```python
from build123d import *

# Parameters (mm, degrees)
MODEL_R             = 95.25
MODEL_R_2           = 85.725
MODEL_R_3           = 1.6724
BOSS_EXTRUDE1_DEPTH = 4


with BuildPart() as part:
    # Model → Boss-Extrude1 (new body)
    with BuildSketch(Plane.XY):
        Circle(MODEL_R)
        Circle(MODEL_R_2, mode=Mode.SUBTRACT)
        with Locations((90.208557236, -7.099567425)):
            Circle(MODEL_R_3, mode=Mode.SUBTRACT)
        with Locations((89.37344872, -14.155363655)):
            Circle(MODEL_R_3, mode=Mode.SUBTRACT)
        with Locations((87.987323172, -21.123887362)):
            Circle(MODEL_R_3, mode=Mode.SUBTRACT)
        with Locations((86.058726518, -27.962175279)):
            Circle(MODEL_R_3, mode=Mode.SUBTRACT)
        with Locations((83.599549198, -34.628067086)):
            Circle(MODEL_R_3, mode=Mode.SUBTRACT)
        with Locations((80.624952857, -41.080465345)):
            Circle(MODEL_R_3, mode=Mode.SUBTRACT)
        with Locations((77.153276872, -47.279588875)):
            Circle(MODEL_R_3, mode=Mode.SUBTRACT)
        with Locations((73.205925279, -53.187218017)):
            Circle(MODEL_R_3, mode=Mode.SUBTRACT)
        with Locations((68.807234812, -58.766930273)):
            Circle(MODEL_R_3, mode=Mode.SUBTRACT)
        with Locations((63.984324863, -63.984324863)):
            Circle(MODEL_R_3, mode=Mode.SUBTRACT)
        with Locations((58.766930273, -68.807234812)):
            Circle(MODEL_R_3, mode=Mode.SUBTRACT)
        with Locations((53.187218017, -73.205925279)):
            Circle(MODEL_R_3, mode=Mode.SUBTRACT)
        with Locations((47.279588875, -77.153276872)):
            Circle(MODEL_R_3, mode=Mode.SUBTRACT)
        with Locations((41.080465345, -80.624952857)):
            Circle(MODEL_R_3, mode=Mode.SUBTRACT)
        with Locations((34.628067086, -83.599549198)):
            Circle(MODEL_R_3, mode=Mode.SUBTRACT)
        with Locations((27.962175279, -86.058726518)):
            Circle(MODEL_R_3, mode=Mode.SUBTRACT)
        with Locations((21.123887362, -87.987323172)):
            Circle(MODEL_R_3, mode=Mode.SUBTRACT)
        with Locations((14.155363655, -89.37344872)):
            Circle(MODEL_R_3, mode=Mode.SUBTRACT)
        with Locations((7.099567425, -90.208557236)):
            Circle(MODEL_R_3, mode=Mode.SUBTRACT)
        with Locations((0, -90.4875)):
            Circle(MODEL_R_3, mode=Mode.SUBTRACT)
        with Locations((-7.099567425, -90.208557236)):
            Circle(MODEL_R_3, mode=Mode.SUBTRACT)
        with Locations((-14.155363655, -89.37344872)):
            Circle(MODEL_R_3, mode=Mode.SUBTRACT)
        with Locations((-21.123887362, -87.987323172)):
            Circle(MODEL_R_3, mode=Mode.SUBTRACT)
        with Locations((-27.962175279, -86.058726518)):
            Circle(MODEL_R_3, mode=Mode.SUBTRACT)
        with Locations((-34.628067086, -83.599549198)):
            Circle(MODEL_R_3, mode=Mode.SUBTRACT)
        with Locations((-41.080465345, -80.624952857)):
            Circle(MODEL_R_3, mode=Mode.SUBTRACT)
        with Locations((-47.279588875, -77.153276872)):
            Circle(MODEL_R_3, mode=Mode.SUBTRACT)
        with Locations((-53.187218017, -73.205925279)):
            Circle(MODEL_R_3, mode=Mode.SUBTRACT)
        with Locations((-58.766930273, -68.807234812)):
            Circle(MODEL_R_3, mode=Mode.SUBTRACT)
        with Locations((-63.984324863, -63.984324863)):
            Circle(MODEL_R_3, mode=Mode.SUBTRACT)
        with Locations((-68.807234812, -58.766930273)):
            Circle(MODEL_R_3, mode=Mode.SUBTRACT)
        with Locations((-73.205925279, -53.187218017)):
            Circle(MODEL_R_3, mode=Mode.SUBTRACT)
        with Locations((-77.153276872, -47.279588875)):
            Circle(MODEL_R_3, mode=Mode.SUBTRACT)
        with Locations((-80.624952857, -41.080465345)):
            Circle(MODEL_R_3, mode=Mode.SUBTRACT)
        with Locations((-83.599549198, -34.628067086)):
            Circle(MODEL_R_3, mode=Mode.SUBTRACT)
        with Locations((-86.058726518, -27.962175279)):
            Circle(MODEL_R_3, mode=Mode.SUBTRACT)
        with Locations((-87.987323172, -21.123887362)):
            Circle(MODEL_R_3, mode=Mode.SUBTRACT)
        with Locations((-89.37344872, -14.155363655)):
            Circle(MODEL_R_3, mode=Mode.SUBTRACT)
        with Locations((-90.208557236, -7.099567425)):
            Circle(MODEL_R_3, mode=Mode.SUBTRACT)
        with Locations((-90.4875, 0)):
            Circle(MODEL_R_3, mode=Mode.SUBTRACT)
        with Locations((-90.208557236, 7.099567425)):
            Circle(MODEL_R_3, mode=Mode.SUBTRACT)
        with Locations((-89.37344872, 14.155363655)):
            Circle(MODEL_R_3, mode=Mode.SUBTRACT)
        with Locations((-87.987323172, 21.123887362)):
            Circle(MODEL_R_3, mode=Mode.SUBTRACT)
        with Locations((-86.058726518, 27.962175279)):
            Circle(MODEL_R_3, mode=Mode.SUBTRACT)
        with Locations((-83.599549198, 34.628067086)):
            Circle(MODEL_R_3, mode=Mode.SUBTRACT)
        with Locations((-80.624952857, 41.080465345)):
            Circle(MODEL_R_3, mode=Mode.SUBTRACT)
        with Locations((-77.153276872, 47.279588875)):
            Circle(MODEL_R_3, mode=Mode.SUBTRACT)
        with Locations((-73.205925279, 53.187218017)):
            Circle(MODEL_R_3, mode=Mode.SUBTRACT)
        with Locations((-68.807234812, 58.766930273)):
            Circle(MODEL_R_3, mode=Mode.SUBTRACT)
        with Locations((-63.984324863, 63.984324863)):
            Circle(MODEL_R_3, mode=Mode.SUBTRACT)
        with Locations((-58.766930273, 68.807234812)):
            Circle(MODEL_R_3, mode=Mode.SUBTRACT)
        with Locations((-53.187218017, 73.205925279)):
            Circle(MODEL_R_3, mode=Mode.SUBTRACT)
        with Locations((-47.279588875, 77.153276872)):
            Circle(MODEL_R_3, mode=Mode.SUBTRACT)
        with Locations((-41.080465345, 80.624952857)):
            Circle(MODEL_R_3, mode=Mode.SUBTRACT)
        with Locations((-34.628067086, 83.599549198)):
            Circle(MODEL_R_3, mode=Mode.SUBTRACT)
        with Locations((-27.962175279, 86.058726518)):
            Circle(MODEL_R_3, mode=Mode.SUBTRACT)
        with Locations((-21.123887362, 87.987323172)):
            Circle(MODEL_R_3, mode=Mode.SUBTRACT)
        with Locations((-14.155363655, 89.37344872)):
            Circle(MODEL_R_3, mode=Mode.SUBTRACT)
        with Locations((-7.099567425, 90.208557236)):
            Circle(MODEL_R_3, mode=Mode.SUBTRACT)
        with Locations((0, 90.4875)):
            Circle(MODEL_R_3, mode=Mode.SUBTRACT)
        with Locations((7.099567425, 90.208557236)):
            Circle(MODEL_R_3, mode=Mode.SUBTRACT)
        with Locations((14.155363655, 89.37344872)):
            Circle(MODEL_R_3, mode=Mode.SUBTRACT)
        with Locations((21.123887362, 87.987323172)):
            Circle(MODEL_R_3, mode=Mode.SUBTRACT)
        with Locations((27.962175279, 86.058726518)):
            Circle(MODEL_R_3, mode=Mode.SUBTRACT)
        with Locations((34.628067086, 83.599549198)):
            Circle(MODEL_R_3, mode=Mode.SUBTRACT)
        with Locations((41.080465345, 80.624952857)):
            Circle(MODEL_R_3, mode=Mode.SUBTRACT)
        with Locations((47.279588875, 77.153276872)):
            Circle(MODEL_R_3, mode=Mode.SUBTRACT)
        with Locations((53.187218017, 73.205925279)):
            Circle(MODEL_R_3, mode=Mode.SUBTRACT)
        with Locations((58.766930273, 68.807234812)):
            Circle(MODEL_R_3, mode=Mode.SUBTRACT)
        with Locations((63.984324863, 63.984324863)):
            Circle(MODEL_R_3, mode=Mode.SUBTRACT)
        with Locations((68.807234812, 58.766930273)):
            Circle(MODEL_R_3, mode=Mode.SUBTRACT)
        with Locations((73.205925279, 53.187218017)):
            Circle(MODEL_R_3, mode=Mode.SUBTRACT)
        with Locations((77.153276872, 47.279588875)):
            Circle(MODEL_R_3, mode=Mode.SUBTRACT)
        with Locations((80.624952857, 41.080465345)):
            Circle(MODEL_R_3, mode=Mode.SUBTRACT)
        with Locations((83.599549198, 34.628067086)):
            Circle(MODEL_R_3, mode=Mode.SUBTRACT)
        with Locations((86.058726518, 27.962175279)):
            Circle(MODEL_R_3, mode=Mode.SUBTRACT)
        with Locations((87.987323172, 21.123887362)):
            Circle(MODEL_R_3, mode=Mode.SUBTRACT)
        with Locations((89.37344872, 14.155363655)):
            Circle(MODEL_R_3, mode=Mode.SUBTRACT)
        with Locations((90.208557236, 7.099567425)):
            Circle(MODEL_R_3, mode=Mode.SUBTRACT)
        with Locations((90.4875, 0)):
            Circle(MODEL_R_3, mode=Mode.SUBTRACT)
    extrude(amount=BOSS_EXTRUDE1_DEPTH)


solid = part.part
```
Here's how the part is built. I have some questions about the finished solid (model axes, mm). Coordinates: 2 decimals unless noted, no trailing zeros. Return JSON: item names as keys, results as strings.
1) I need wall thicknesses on line 1 (Y direction, x = 27, z = 2.3); line 2 (X direction, y = -78.5, z = 2.95); line 3 (Y direction, x = -46, z = 1.1). Which ranges of each line are inside material? Lowest first, please. Write a range as from..to.
Results below:
{"line 1": "-91.34..-87.43, -84.69..-81.36, 81.36..84.69, 87.43..91.34", "line 2": "-53.95..-48.27, -46.29..-34.45, 34.45..46.29, 48.27..53.95", "line 3": "-83.41..-78.23, -76.08..-72.34, 72.34..76.08, 78.23..83.41"}
2) Will these pins go through, and if not, where does the flat tip stop? pin 1 (1 mm diameter, centred on y = -65, z = 3.5, fed in from -X); pin 2 (4 mm diameter, centred on x = -73.21, y = -53.19, fed in from -Z); pin 3 (2 mm diameter, centred on y = -18.5, z = 2, fed in from +X); pin 4 (1.5 mm diameter, centred on y = 51.5, z = 2, fed in from -X).
Results below:
{"pin 1": "x = -70.09", "pin 2": "z = 0", "pin 3": "x = 93.63", "pin 4": "x = -80.6"}
3) If we section it at A-A, the plane z = 1.75: Count the separate pieces of the cut face and the enclosed holes in it, then the cut area to 3 significant figures.
Results below:
{"separate pieces": "1", "enclosed holes": "81", "area": "4,710 mm²"}
4) Thinking about a two-plate mould opening in Y: for faces 1 (the face through (-78, 36, 0)), 2 (the face through (46.09, 72.28, 1.97)), 3 (the face through (-75.587, -57.958, 1.972)), which applies, +Y half, -Y half, draft (parallel to the pull), parting line (faces both ways), or undercut?
Results below:
{"face 1": "draft", "face 2": "undercut", "face 3": "parting line"}
